```python
from build123d import *

# Parameters (mm, degrees)
BOSS_EXTRUDE1_DEPTH = 4
SKETCH3_W           = 3
SKETCH3_H           = 30
BOSS_EXTRUDE2_DEPTH = 30
BOSS_EXTRUDE3_DEPTH = 4
CHAMFER1_SIZE       = 5
CHAMFER2_SIZE       = 5
CHAMFER3_SIZE       = 1
CUT_EXTRUDE3_REACH  = 5
SKETCH6_R           = 1.55
CUT_EXTRUDE4_REACH  = 6
SKETCH7_R           = 2.4
CUT_EXTRUDE5_REACH  = 6
SKETCH8_R           = 0.5


with BuildPart() as part:
    # Sketch1 → Boss-Extrude1 (new body)
    with BuildSketch(Plane.XY):
        with BuildLine():
            Line((-24.444, 20.55625), (-24.444, -9.44375))
            Line((-24.444, -9.44375), (-21.444, -9.44375))
            Line((-21.444, -9.44375), (7.320666414, -4.286816212))
            ThreePointArc((7.320666414, -4.286816212), (15.556, 5.55625), (7.320666414, 15.399316212))
            Line((7.320666414, 15.399316212), (-21.444, 20.55625))
            Line((-21.444, 20.55625), (-24.444, 20.55625))
        make_face()
    extrude(amount=BOSS_EXTRUDE1_DEPTH)

    # Sketch3 → Boss-Extrude2 (add)
    with BuildSketch(Plane(origin=(0, 0, 0), x_dir=(-1, 0, 0), z_dir=(0, 0, -1))):
        with Locations((22.944, 5.55625)):
            Rectangle(SKETCH3_W, SKETCH3_H)
    extrude(amount=BOSS_EXTRUDE2_DEPTH)

    # Sketch4 → Boss-Extrude3 (add)
    with BuildSketch(Plane(origin=(2.902788428, 16.191354052, 0), x_dir=(0.984306621, -0.176466641, 0), z_dir=(0.176466641, 0.984306621, 0))):
        Polygon((-24.734963581, 22.5), (-10.123324385, 0), (-10.123324385, -0.5), (-24.734963581, -0.5), align=None)
    extrude(amount=-BOSS_EXTRUDE3_DEPTH)

    # Chamfer1
    chamfer1_edges = [part.edges().sort_by_distance(p)[0] for p in [
        (-21.444, 3.524362825, 0),
    ]]
    chamfer(chamfer1_edges, length=CHAMFER1_SIZE)

    # Chamfer2
    chamfer2_edges = [part.edges().sort_by_distance(p)[0] for p in [
        (-22.944, 20.55625, -30),
        (-22.944, -9.44375, -30),
    ]]
    chamfer(chamfer2_edges, length=CHAMFER2_SIZE)

    # Chamfer3
    chamfer3_edges = [part.edges().sort_by_distance(p)[0] for p in [
        (-7.061666793, -6.865283106, 4),
        (15.556, 5.55625, 4),
        (-7.061666793, 17.977783106, 4),
    ]]
    chamfer(chamfer3_edges, length=CHAMFER3_SIZE)

    # Sketch6 → Cut-Extrude3 (cut, up to next)
    with BuildSketch(Plane(origin=(-21.444, 0, 0), x_dir=(0, 0, -1), z_dir=(1, 0, 0)), mode=Mode.PRIVATE) as cut_extrude3_sk1:
        with Locations((11, 9.04722098)):
            Circle(SKETCH6_R)
    cut_extrude3_tool1 = extrude(cut_extrude3_sk1.sketch, amount=-CUT_EXTRUDE3_REACH, mode=Mode.PRIVATE) & part.part
    add(cut_extrude3_tool1.solids().sort_by_distance((-21.444, 9.047221, -11))[0], mode=Mode.SUBTRACT)
    # Sketch6 → Cut-Extrude3 (cut, up to next)
    with BuildSketch(Plane(origin=(-21.444, 0, 0), x_dir=(0, 0, -1), z_dir=(1, 0, 0)), mode=Mode.PRIVATE) as cut_extrude3_sk2:
        with Locations((24, 9.04722098)):
            Circle(SKETCH6_R)
    cut_extrude3_tool2 = extrude(cut_extrude3_sk2.sketch, amount=-CUT_EXTRUDE3_REACH, mode=Mode.PRIVATE) & part.part
    add(cut_extrude3_tool2.solids().sort_by_distance((-21.444, 9.047221, -24))[0], mode=Mode.SUBTRACT)
    # Sketch6 → Cut-Extrude3 (cut, up to next)
    with BuildSketch(Plane(origin=(-21.444, 0, 0), x_dir=(0, 0, -1), z_dir=(1, 0, 0)), mode=Mode.PRIVATE) as cut_extrude3_sk3:
        with Locations((11, -1.889802378)):
            Circle(SKETCH6_R)
    cut_extrude3_tool3 = extrude(cut_extrude3_sk3.sketch, amount=-CUT_EXTRUDE3_REACH, mode=Mode.PRIVATE) & part.part
    add(cut_extrude3_tool3.solids().sort_by_distance((-21.444, -1.889802, -11))[0], mode=Mode.SUBTRACT)
    # Sketch6 → Cut-Extrude3 (cut, up to next)
    with BuildSketch(Plane(origin=(-21.444, 0, 0), x_dir=(0, 0, -1), z_dir=(1, 0, 0)), mode=Mode.PRIVATE) as cut_extrude3_sk4:
        with Locations((24, -1.889802378)):
            Circle(SKETCH6_R)
    cut_extrude3_tool4 = extrude(cut_extrude3_sk4.sketch, amount=-CUT_EXTRUDE3_REACH, mode=Mode.PRIVATE) & part.part
    add(cut_extrude3_tool4.solids().sort_by_distance((-21.444, -1.889802, -24))[0], mode=Mode.SUBTRACT)

    # Sketch7 → Cut-Extrude4 (cut, up to next)
    with BuildSketch(Plane(origin=(0, 0, 0), x_dir=(-1, 0, 0), z_dir=(0, 0, -1)), mode=Mode.PRIVATE) as cut_extrude4_sk1:
        with Locations((-5.556, 5.55625)):
            Circle(SKETCH7_R)
    cut_extrude4_tool1 = extrude(cut_extrude4_sk1.sketch, amount=-CUT_EXTRUDE4_REACH, mode=Mode.PRIVATE) & part.part
    add(cut_extrude4_tool1.solids().sort_by_distance((5.556, 5.55625, 0))[0], mode=Mode.SUBTRACT)

    # Sketch8 → Cut-Extrude5 (cut, up to next)
    with BuildSketch(Plane(origin=(0, 0, 0), x_dir=(-1, 0, 0), z_dir=(0, 0, -1)), mode=Mode.PRIVATE) as cut_extrude5_sk1:
        with Locations((9.444, 5.55625)):
            Circle(SKETCH8_R)
    cut_extrude5_tool1 = extrude(cut_extrude5_sk1.sketch, amount=-CUT_EXTRUDE5_REACH, mode=Mode.PRIVATE) & part.part
    add(cut_extrude5_tool1.solids().sort_by_distance((-9.444, 5.55625, 0))[0], mode=Mode.SUBTRACT)
    # Sketch8 → Cut-Extrude5 (cut, up to next)
    with BuildSketch(Plane(origin=(0, 0, 0), x_dir=(-1, 0, 0), z_dir=(0, 0, -1)), mode=Mode.PRIVATE) as cut_extrude5_sk2:
        with Locations((-5.556, 11.65625)):
            Circle(SKETCH8_R)
    cut_extrude5_tool2 = extrude(cut_extrude5_sk2.sketch, amount=-CUT_EXTRUDE5_REACH, mode=Mode.PRIVATE) & part.part
    add(cut_extrude5_tool2.solids().sort_by_distance((5.556, 11.65625, 0))[0], mode=Mode.SUBTRACT)
    # Sketch8 → Cut-Extrude5 (cut, up to next)
    with BuildSketch(Plane(origin=(0, 0, 0), x_dir=(-1, 0, 0), z_dir=(0, 0, -1)), mode=Mode.PRIVATE) as cut_extrude5_sk3:
        with Locations((-5.556, -0.54375)):
            Circle(SKETCH8_R)
    cut_extrude5_tool3 = extrude(cut_extrude5_sk3.sketch, amount=-CUT_EXTRUDE5_REACH, mode=Mode.PRIVATE) & part.part
    add(cut_extrude5_tool3.solids().sort_by_distance((5.556, -0.54375, 0))[0], mode=Mode.SUBTRACT)
    # Sketch8 → Cut-Extrude5 (cut, up to next)
    with BuildSketch(Plane(origin=(0, 0, 0), x_dir=(-1, 0, 0), z_dir=(0, 0, -1)), mode=Mode.PRIVATE) as cut_extrude5_sk4:
        with Locations((-12.056, 5.55625)):
            Circle(SKETCH8_R)
    cut_extrude5_tool4 = extrude(cut_extrude5_sk4.sketch, amount=-CUT_EXTRUDE5_REACH, mode=Mode.PRIVATE) & part.part
    add(cut_extrude5_tool4.solids().sort_by_distance((12.056, 5.55625, 0))[0], mode=Mode.SUBTRACT)


solid = part.part
```
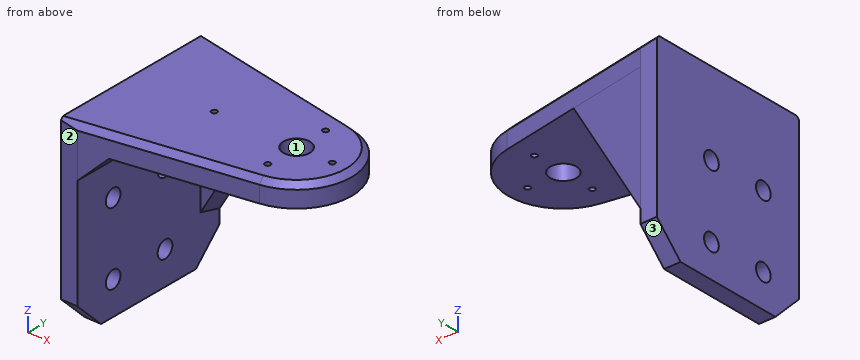
Source: CAD feature listing. Evaluate the final solid. Frame: model axes, mm. Face numbers are marked on the shaded views. Coordinates: 2 decimals unless noted, no trailing zeros. Write each loop counter-clockwise with the first axis right and the second up, starting at its lowest first coordinate (ties: lowest second). Pieces come first, ordered by that corner, then holes. Notation, with made-up numbers: (51.5, -12) - (60.5, -12) arc R29 ccw to (60.5, 21) - close; hole circle Ø8 at (12, 29.5). An arc over 180 degrees is marked (long way). Answer as a JSON object with one key per item and string values.
Q1. Section query B-B, the plane y = -7.5. Output: boundary loops of the cut face in (x, z).
Ans:
{"outline": "(-24.44, -26.94) - (-21.44, -26.94) - (-21.44, -5) - (-16.44, 0) - (-10.6, 0) - (-10.6, 3) - (-16.27, 4) - (-24.44, 4) - close"}
Q2. First-contact query: pin 1 Ø1 at (x, y) = (7.5, 11) entering from -Z; pin 2 Ø7.5 at (y, z) = (1, -21.5) entering from +X; pin 3 Ø1.5 at (y, z) = (0, -4.5) entering from +X. Flat tips, straight axial feed; report the tip coordinate or a pass-through.
Ans:
{"pin 1": "stops at z = 0", "pin 2": "stops at x = -21.44", "pin 3": "stops at x = -20.19"}
Q3. Draft query along Y for the marked faces 1, 2 and 3. Return one class per face: released by +Y, released by -Y, zero draft, split by the parting line, or undercut.
Ans:
{"face 1": "undercut", "face 2": "released by -Y", "face 3": "released by +Y"}
Q4. Section query A-A, the plane z = -24. Output: boundary loops of the cut face in (x, y), plus the area to 3 significant figures.
Ans:
{"outline": "(-24.44, -9.44) - (-21.44, -9.44) - (-21.44, -3.44) - (-24.44, -3.44) - close; (-24.44, -0.34) - (-21.44, -0.34) - (-21.44, 7.5) - (-24.44, 7.5) - close; (-24.44, 10.6) - (-21.44, 10.6) - (-21.44, 20.56) - (-24.44, 20.56) - close", "area": "71.4 mm2"}
Q5. Section query C-C, the plane z = -2.5. Output: boundary loops of the cut face in (x, y).
Ans:
{"outline": "(-24.44, -9.44) - (-21.44, -9.44) - (-18.94, -9) - (-18.94, 16.04) - (-9.37, 14.33) - (-8.66, 18.26) - (-21.44, 20.56) - (-24.44, 20.56) - close"}
Q6. Material intervals for line 1 (Y direction, x = -22.9, z = -11); line 2 (X direction, y = 3.75, z = -22); line 3 (Z direction, x = 12, y = 7), sorted ascending. Write a range as [from, to].
Ans:
{"line 1": "y = [-9.44, -3.44], [-0.34, 7.5], [10.6, 20.56]", "line 2": "x = [-24.44, -21.44]", "line 3": "z = [0, 4]"}
Q7. Section query D-D, the plane z = -11. Output: boundary loops of the cut face in (x, y), plus the area to 3 significant figures.
Ans:
{"outline": "(-24.44, -9.44) - (-21.44, -9.44) - (-21.44, -3.44) - (-24.44, -3.44) - close; (-24.44, -0.34) - (-21.44, -0.34) - (-21.44, 7.5) - (-24.44, 7.5) - close; (-24.44, 10.6) - (-21.44, 10.6) - (-21.44, 16.49) - (-14.8, 15.3) - (-14.09, 19.24) - (-21.44, 20.56) - (-24.44, 20.56) - close", "area": "99.8 mm2"}
